```python
from build123d import *

# Parameters (mm, degrees)
SKETCH1_R           = 1.143
SKETCH1_R_2         = 5.033023
BOSS_EXTRUDE1_DEPTH = 2.54
SKETCH2_R           = 5.033023
BOSS_EXTRUDE2_DEPTH = 2.54


with BuildPart() as part:
    # Sketch1 → Boss-Extrude1 (new body)
    with BuildSketch(Plane.XY):
        with BuildLine():
            Line((-2.758484, 1.414769), (-5.574053, -0.790422))
            ThreePointArc((-5.574053, -0.790422), (-8.368053, -3.584422), (-5.574053, -6.378422))
            Line((-5.574053, -6.378422), (-2.892677, -8.47851))
            ThreePointArc((-2.892677, -8.47851), (1.156947, -9.936709), (5.20657, -8.47851))
            Line((5.20657, -8.47851), (7.887947, -6.378422))
            ThreePointArc((7.887947, -6.378422), (10.681947, -3.584422), (7.887947, -0.790422))
            Line((7.887947, -0.790422), (5.20657, 1.309667))
            ThreePointArc((5.20657, 1.309667), (1.3274, 2.765578), (-2.62429, 1.519871))
            Line((-2.62429, 1.519871), (-2.758484, 1.414769))
        make_face()
        with Locations((7.887947, -3.584422)):
            Circle(SKETCH1_R, mode=Mode.SUBTRACT)
        with Locations((-5.574053, -3.584422)):
            Circle(SKETCH1_R, mode=Mode.SUBTRACT)
        with Locations((1.156947, -3.584422)):
            Circle(SKETCH1_R_2, mode=Mode.SUBTRACT)
    extrude(amount=BOSS_EXTRUDE1_DEPTH)

    # Sketch2 → Boss-Extrude2 (add)
    with BuildSketch(Plane(origin=(0, 0, 0), x_dir=(-1, 0, 0), z_dir=(0, 0, -1))):
        with BuildLine():
            ThreePointArc((5.106789, -2.541295), (-1.156947, 2.765578), (-7.420683, -2.541295))
            ThreePointArc((-7.420683, -2.541295), (-6.744947, -3.584422), (-7.420683, -4.627548))
            ThreePointArc((-7.420683, -4.627548), (-1.156947, -9.934422), (5.106789, -4.627548))
            ThreePointArc((5.106789, -4.627548), (4.431053, -3.584422), (5.106789, -2.541295))
        make_face()
        with Locations((-1.156947, -3.584422)):
            Circle(SKETCH2_R, mode=Mode.SUBTRACT)
    extrude(amount=BOSS_EXTRUDE2_DEPTH)

    # Sketch5 → Revolve1 (revolve)
    with BuildSketch(Plane(origin=(1.156947, 0, 0), x_dir=(0, 0, -1), z_dir=(1, 0, 0))):
        with BuildLine():
            Line((2.54, -3.584422), (7.62, -3.584422))
            ThreePointArc((7.62, -3.584422), (6.132102, 0.007681), (2.54, 1.495578))
            Line((2.54, 1.495578), (2.54, -3.584422))
        make_face()
    revolve(axis=Axis((1.156947, -3.584422, -2.54), (0, 0, -1)))


solid = part.part
```
Design review of the part built by this model. Coordinates are the model's own, in mm. A direction names the side the tool comes from. Give positions to 0.01 mm unless a question says otherwise; leave off trailing zeros. Loops run counter-clockwise (first coordinate to the right, second up) from the corner with the lowest first, then second, coordinate; pieces in that order, holes last. Notation, with made-up numbers: M 27,-13 L 36,-13 A13 cw 36,0 Z; hole C 37.5,41.25 d8. An arc over 180 degrees is marked long. Return JSON: item names as keys, results as strings. Group by question number.
Item 1: Mouldability with a two-part tool opening along X and no side actions: class faces 1 (the flat face through (-4.252, -7.414, 1.252)), 2 (the flat face through (1, -4, -2.54)), 3 (the flat face through (6.57, 0.24, 1.25)) as released by +X, released by -X, zero draft, split by the parting line, or undercut.
Item 2: For probe 1 along X at (y, z) = (-3.5, 1.75); probe 2 along Z at (x, y) = (9.75, -3.75); probe 3 along Y at (x, z) = (-2, 0), list the stretches that pass through material, from the lowest coordinate up.
Item 3: We need section B-B (z = 1.75). Give the boundary of the cut face in (x, y).
Item 4: We need section C-C (y = -3). Give the number of separate pieces and of enclosed holes in the cut face, and give its area (3 significant figures).
Item 5: Insertion check: pin 1 Ø5 at (x, y) = (5.5, -6.5) entering from -Z; pin 2 Ø2 at (x, z) = (1, -2) entering from +Y; pin 3 Ø2.5 at (x, y) = (-5.57, -3.58) entering from +Z; pin 4 Ø3 at (x, y) = (7.89, -3.58) entering from -Z. Each pin has a flat end and moves straight along its axis. Give the tip position at first contact, or say it passes through.
Item 6: We need section A-A (x = 8.75). Give the boundary of the cut face in (y, z), and give its area (3 significant figures).
Item 7: Tool access review of faces 4 (the cylindrical face through (1.095, -9.936, 1.252)), 5 (the flat face through (6.53, -7.44, 1.25)), 6 (the cylindrical face through (1.032, 2.764, -1.252)), 7 (the cylindrical face through (1.282, -9.933, -1.252)), 8 (the flat face through (4, 1, -2.54)): name each direction out of +Z, -Z, +X, -X, +Y, -Y from which nothing blocks a thin tool from reaching the whole face with its end or side.
Output:
{
 "1": {"face 1": "released by -X", "face 2": "undercut", "face 3": "released by +X"},
 "2": {"probe 1": "x = -8.37 to -6.71, -4.43 to -3.88, 6.19 to 6.75, 9.03 to 10.68", "probe 2": "z = 0 to 2.54", "probe 3": "y = -9.09 to -7.5, 0.34 to 1.93"},
 "3": {"outline": "M -5.57,-6.38 L -2.89,-8.48 A6.35 ccw 5.21,-8.48 L 7.89,-6.38 A2.79 ccw 7.89,-0.79 L 5.21,1.31 A6.35 ccw -2.62,1.52 L -2.76,1.41 L -5.57,-0.79 A2.79 ccw Z; hole C -5.57,-3.58 d2.29; hole C 1.16,-3.58 d10.07; hole C 7.89,-3.58 d2.29"},
 "4": {"separate pieces": "3", "enclosed holes": "0", "area": "56.5 mm^2"},
 "5": {"pin 1": "stops at z = -6.82", "pin 2": "stops at y = 2.77", "pin 3": "stops at z = 2.54", "pin 4": "stops at z = -2.54"},
 "6": {"outline": "M -6.24,0 L -4.33,0 L -4.33,2.54 L -6.24,2.54 Z; M -2.83,0 L -0.93,0 L -0.93,2.54 L -2.83,2.54 Z", "area": "9.69 mm^2"},
 "7": {"face 4": "+Z, -Z, -Y", "face 5": "+Z, -Z, +X, -Y", "face 6": "-Z, +Y", "face 7": "-Z, -Y", "face 8": "-Z"}
}
